```python
from build123d import *

# Parameters (mm, degrees)
BASPROSKE_W     = 12.7
BASPROSKE_H     = 7.9375
TOOTHCUT_DEPTH  = 17.949861725
TEETHCUTS_COUNT = 18
TEETHCUTS_ANGLE = 340
BORSKE_R        = 3
BORE_DEPTH      = 50.8000508


with BuildPart() as part:
    # BasProSke → Base-Revolve (revolve)
    with BuildSketch(Plane(origin=(0, 0, 0), x_dir=(1, 0, 0), z_dir=(0, 1, 0)), mode=Mode.PRIVATE) as base_revolve_sk:
        with Locations((6.35, 3.96875)):
            Rectangle(BASPROSKE_W, BASPROSKE_H)
    revolve(base_revolve_sk.sketch.rotate(Axis((-10, 0, 0), (1, 0, 0)), 180), axis=Axis((-10, 0, 0), (1, 0, 0)))

    # TooCutSke → ToothCut (cut, through all)
    with BuildSketch(Plane(origin=(0, 0, 0), x_dir=(0, 0, -1), z_dir=(1, 0, 0))):
        with BuildLine():
            ThreePointArc((0.401805019, 6.127289689), (0, 6.14045), (-0.401805019, 6.127289689))
            ThreePointArc((-0.401805019, 6.127289689), (-0.651999955, 7.068698885), (-1.203877601, 7.87136933))
            ThreePointArc((-1.203877601, 7.87136933), (0, 7.9629), (1.203877601, 7.87136933))
            ThreePointArc((1.203877601, 7.87136933), (0.651999955, 7.068698885), (0.401805019, 6.127289689))
        make_face()
    toothcut = extrude(amount=TOOTHCUT_DEPTH, mode=Mode.SUBTRACT)

    # TeethCuts: ToothCut ×18 about axis
    teethcuts_axis = Axis((-10, 0, 0), (1, 0, 0))
    for i in range(1, TEETHCUTS_COUNT):
        add(toothcut.rotate(teethcuts_axis, i * TEETHCUTS_ANGLE / (TEETHCUTS_COUNT - 1)), mode=Mode.SUBTRACT)

    # BorSke → Bore (cut, symmetric)
    with BuildSketch(Plane(origin=(0, 0, 0), x_dir=(0, 0, -1), z_dir=(1, 0, 0))):
        with Locations(Location((0, 0, 0), (0, 0, 180))):
            Circle(BORSKE_R)
    extrude(amount=BORE_DEPTH, both=True, mode=Mode.SUBTRACT)

    # Sketch1 → Revolve1 (revolve)
    with BuildSketch(Plane.XY, mode=Mode.PRIVATE) as revolve1_sk:
        Polygon((12.7, 6.14045), (17.65, 6.46), (17.65, 4.46), (12.7, 4.46), align=None)
    revolve(revolve1_sk.sketch.rotate(Axis((12.7, 0, 0), (1, 0, 0)), 180), axis=Axis((12.7, 0, 0), (1, 0, 0)))


solid = part.part
```
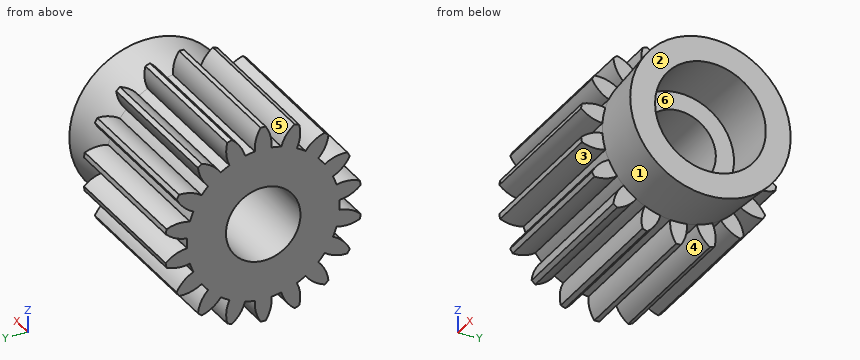
Work out the finished part from the listing and answer in its coordinate system (mm). Face numbers are marked on the shaded views. A direction names the side the tool comes from. Round coordinates to 2 decimals unless told otherwise and drop trailing zeros. Loops run counter-clockwise (first coordinate to the right, second up) from the corner with the lowest first, then second, coordinate; pieces in that order, holes last. Notation, with made-up numbers: M 69,-17.75 L 78,-17.75 A20 ccw 78,6.25 Z; hole C 77.5,32.25 d4. An arc over 180 degrees is marked long. Use CSV: the item, a comma, the result in double quotes.
Q1. A tool of negligible diameter and unlimited length cuts with its end or side. For the marked faces 4, 5 and 6, from which of +Z, -Z, +X, -X, +Y, -Y can it reach the whole face along a straight path? Write none if from no direction.
Determined:
face 4,"-Z, -X"
face 5,"+Z, -X"
face 6,"+X"
Q2. Each of these flat-tipped pins is pushed along its axis until it touches: pin 1 (0.5 mm diameter, centred on y = 6.5, z = 3, fed in from +X); pin 2 (4 mm diameter, centred on x = 15, y = -5, fed in from +Z); pin 3 (6 mm diameter, centred on x = 9, y = -4, fed in from -Z). Where does it stop, or does it pass through?
Determined:
pin 1,"x = 12.7"
pin 2,"z = 5.54"
pin 3,"z = -7.52"
Q3. Consider L1, parallel to Y at x = 10.25, z = 0; L2, parallel to Z at x = 13.8, y = 0; L3, parallel to Y at x = 12.5, z = 6.5. Determine where each line is inside the solid, lowest interval first.
Determined:
L1,"-6.14 to -3, 3 to 6.14"
L2,"-6.21 to -4.46, 4.46 to 6.21"
L3,"-2.97 to -1.66, -0.67 to 0.67, 1.66 to 2.97"
Q4. Section B-B, the plane z = 6.75 is taken. Determine the outline of the cut face in (x, y).
Determined:
outline,"M 0,-2.98 L 12.7,-2.98 L 12.7,-1.8 L 0,-1.8 Z; M 0,-0.65 L 12.7,-0.65 L 12.7,0.65 L 0,0.65 Z; M 0,1.8 L 12.7,1.8 L 12.7,2.98 L 0,2.98 Z"
Q5. The mould has two halves that part along Y. Classify the marked faces 1, 2 and 3: pulls with the +Y half, pulls with the -Y half, needs draft (parallel to the pull), parting line crosses it, or undercut.
Determined:
face 1,"parting line crosses it"
face 2,"needs draft"
face 3,"undercut"
Q6. Section A-A, the plane z = 0 is taken. Determine the outline of the cut face in (x, y).
Determined:
outline,"M 0,-6.14 L 12.7,-6.14 L 17.65,-6.46 L 17.65,-4.46 L 12.7,-4.46 L 12.7,-3 L 0,-3 Z; M 0,3 L 12.7,3 L 12.7,4.46 L 17.65,4.46 L 17.65,6.46 L 12.7,6.14 L 0,6.14 Z"
